```python
from build123d import *

# Parameters (mm, degrees)
F0_W     = 107.5221002102
F0_H     = 52.1313343197
F1_DEPTH = 49.57312
F2_W     = 107.5221002102
F2_H     = 26.3976580463
F3_DEPTH = 25.04967
F6_D     = 19.05
F7_D     = 19.05
F7_DEPTH = 12.7
F7_TIP   = 5.7231973962


with BuildPart() as f1:
    # F0 (on Top) → F1 (new body)
    with BuildSketch(Plane.XY):
        with Locations((-0.1560784876, 13.9232939109)):
            Rectangle(F0_W, F0_H)
    extrude(amount=F1_DEPTH)

    # F2 (on face) → F3 (join)
    with BuildSketch(Plane.XY.offset(49.57312)):
        with Locations((-0.1560784876, 17.2676101793)):
            Rectangle(F2_W, F2_H)
    extrude(amount=F3_DEPTH)

    # F6 (through all)
    with Locations(Plane.YZ.offset(53.6049716175)):
        with Locations((14.0758333728, 24.4949776679)):
            Hole(F6_D / 2)

    # F7
    with Locations(Plane.XZ.offset(12.1423732489)):
        with Locations((-32.0040024817, 21.6798111796), (28.5961665213, 21.6798111796)):
            Hole(F7_D / 2, depth=F7_DEPTH)
            with Locations((0, 0, -(F7_DEPTH + F7_TIP / 2))):  # 118° drill point
                Cone(0, F7_D / 2, F7_TIP, mode=Mode.SUBTRACT)


solid = f1.part
```
The listing builds one solid part. Answer for the finished solid, in the listing's coordinates (mm). A direction names the side the tool comes from. Round coordinates to 2 decimals unless told otherwise and drop trailing zeros. Order: outer loops, then holes, each group sorted by start corner. A loop starts at its lowest first (then second) coordinate and runs counter-clockwise, first axis right, second up. Notation, with made-up numbers: (53, 50) -> (67, 50) arc R29 ccw to (67, 86) -> close; hole circle Ø2 at (25.25, 73.5). An arc over 180 degrees is marked (long way). Answer as CSV lines item,"result". Start each with the question number.
(1) The part is cut by section C-C (y = -8.5). Determine the outline of the cut face in (x, z) (3 decimals), then the cut area to 3 significant figures.
(2) The part is cut by section B-B (y = 13). Determine the outline of the cut face in (x, z).
(3) The part is cut by section D-D (z = 62). Determine the outline of the cut face in (x, y), then the cut area to 3 significant figures.
(4) Flat-ended cylindrical pins translate along their axes: pin 1 Ø7.5 at (x, z) = (-3.5, 67) entering from -Y; pin 2 Ø1 at (x, y) = (19, 3.5) entering from +Z. Find the tip coordinate at first contact, or state that the pin passes through.
(5) A tool of negligible diameter and unlimited length cuts with its end or side. For faces 1 (the face through (-1, 35, 49.573)), 2 (the face through (-1, 4.069, 62)), 3 (the face through (-1, 39.989, 24)), 4 (the face through (24.2, -5.7, 13.23)), from which of +Z, -Z, +X, -X, +Y, -Y can it reach the whole face along a straight path? Write none if from no direction.
(6) The part is cut by section A-A (x = -9.5). Determine the outline of the cut face in (y, z) (3 decimals).
(7) For a pull along Z with two mould halves and no side action, classify faces 5 (the face through (29.439, 5.183, 20.059)), 6 (the face through (-0.909, 21.635, 18.699)), 7 (the face through (-1, 17, 74.623)), 8 (the face through (-1, 30.466, 62)) as +Z half, -Z half, draft (parallel to the pull), parting line (faces both ways), or undercut.
(8) Find the intervals of material crossed by probe 1 along Z at (x, y) = (-33, 13.5); probe 2 along Y at (x, z) = (-8, 25); probe 3 along Y at (x, z) = (-17.5, 65.5), in increasing order. Write a range as from..to.
Evaluation:
1,outline,"(-53.917, 0) -> (53.605, 0) -> (53.605, 49.573) -> (-53.917, 49.573) -> close; hole circle Ø19.05 at (-32.004, 21.68); hole circle Ø19.05 at (28.596, 21.68)"
1,area,"4,760 mm²"
2,outline,"(-53.92, 0) -> (53.6, 0) -> (53.6, 15.03) -> (-53.92, 15.03) -> close; (-53.92, 33.96) -> (53.6, 33.96) -> (53.6, 74.62) -> (-53.92, 74.62) -> close"
3,outline,"(-53.92, 4.07) -> (53.6, 4.07) -> (53.6, 30.47) -> (-53.92, 30.47) -> close"
3,area,"2,840 mm²"
4,pin 1,"y = 4.07"
4,pin 2,"z = 49.57"
5,face 1,"+Z, +X, -X, +Y"
5,face 2,"+Z, +X, -X, -Y"
5,face 3,"+Z, -Z, +X, -X, +Y"
5,face 4,"-Y"
6,outline,"(-12.142, 0) -> (39.989, 0) -> (39.989, 49.573) -> (30.466, 49.573) -> (30.466, 74.623) -> (4.069, 74.623) -> (4.069, 49.573) -> (-12.142, 49.573) -> close; hole circle Ø19.05 at (14.076, 24.495)"
7,face 5,"undercut"
7,face 6,"undercut"
7,face 7,"+Z half"
7,face 8,"draft"
8,probe 1,"0..14.99, 34..74.62"
8,probe 2,"-12.14..4.56, 23.59..39.99"
8,probe 3,"4.07..30.47"
